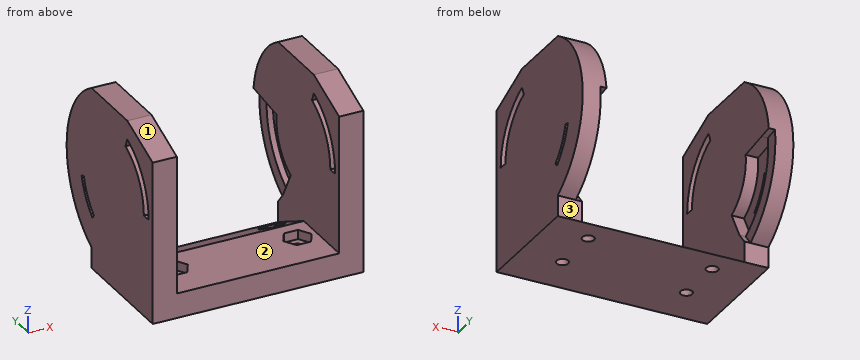
from build123d import *

# Parameters (mm, degrees)
CROQUIS1_W              = 34
CROQUIS1_H              = 19
SALIENTE_EXTRUIR1_DEPTH = 35
CROQUIS2_W              = 26.2
CROQUIS2_H              = 31
CORTAR_EXTRUIR1_DEPTH   = 25
CORTAR_EXTRUIR3_DEPTH   = 26.2
SALIENTE_EXTRUIR2_DEPTH = 34
CROQUIS10_W             = 26.2
CROQUIS10_H             = 25.966324345
CORTAR_EXTRUIR4_DEPTH   = 10
CORTAR_EXTRUIR5_START   = -34
CORTAR_EXTRUIR5_DEPTH   = 34
CORTAR_EXTRUIR6_DEPTH   = 2
CORTAR_EXTRUIR7_START   = 28.2
CORTAR_EXTRUIR7_DEPTH   = 28.2
CORTAR_EXTRUIR8_DEPTH   = 1
CORTAR_EXTRUIR9_DEPTH   = 27.2
CORTAR_EXTRUIR10_START  = -34
CORTAR_EXTRUIR10_DEPTH  = 34
CROQUIS18_R             = 0.95
CORTAR_EXTRUIR11_DEPTH  = 4
CORTAR_EXTRUIR12_DEPTH  = 1.5
CORTAR_EXTRUIR13_DEPTH  = 3


with BuildPart() as part:
    # Croquis1 → Saliente-Extruir1 (new body)
    with BuildSketch(Plane.XY):
        with Locations((-31.887263086, 5.12254902)):
            Rectangle(CROQUIS1_W, CROQUIS1_H)
    extrude(amount=SALIENTE_EXTRUIR1_DEPTH)

    # Croquis2 → Cortar-Extruir1 (cut)
    with BuildSketch(Plane.XZ.offset(4.37745098)):
        with Locations((-31.887263086, 19.5)):
            Rectangle(CROQUIS2_W, CROQUIS2_H)
    extrude(amount=-CORTAR_EXTRUIR1_DEPTH, mode=Mode.SUBTRACT)

    # Croquis4 → Cortar-Extruir3 (cut)
    with BuildSketch(Plane.ZY.offset(18.787263086)):
        Polygon((4, 14.62254902), (4, 6.62254902), (0, 14.62254902), align=None)
    extrude(amount=CORTAR_EXTRUIR3_DEPTH, mode=Mode.SUBTRACT)

    # Croquis9 → Saliente-Extruir2 (add)
    with BuildSketch(Plane(origin=(-14.887263086, 0, 0), x_dir=(0, 0, -1), z_dir=(1, 0, 0))):
        with BuildLine():
            Line((-29.315831827, 14.62254902), (-3.349507482, 14.62254902))
            ThreePointArc((-3.349507482, 14.62254902), (-16.332669655, 22.37254902), (-29.315831827, 14.62254902))
        make_face()
    extrude(amount=-SALIENTE_EXTRUIR2_DEPTH)

    # Croquis10 → Cortar-Extruir4 (cut)
    with BuildSketch(Plane.XZ.offset(-14.62254902)):
        with Locations((-31.887263086, 16.332669655)):
            Rectangle(CROQUIS10_W, CROQUIS10_H)
    extrude(amount=-CORTAR_EXTRUIR4_DEPTH, mode=Mode.SUBTRACT)

    # Croquis11 → Cortar-Extruir5 (cut)
    with BuildSketch(Plane(origin=(-14.887263086, 0, 0), x_dir=(0, 0, -1), z_dir=(1, 0, 0)).offset(CORTAR_EXTRUIR5_START)):
        with BuildLine():
            Line((-26.264575199, 3.509186373), (-24.878727914, 4.083143951))
            ThreePointArc((-24.878727914, 4.083143951), (-21.471881808, -0.068419609), (-16.332669655, -1.62745098))
            Line((-16.332669655, -1.62745098), (-16.332669655, -3.12745098))
            ThreePointArc((-16.332669655, -3.12745098), (-22.305267563, -1.31560371), (-26.264575199, 3.509186373))
        make_face()
        with BuildLine():
            Line((-13.621540157, 17.74062205), (-13.807242822, 17.04757027))
            ThreePointArc((-13.807242822, 17.04757027), (-11.089968726, 15.851941052), (-8.857991001, 13.894549121))
            Line((-8.857991001, 13.894549121), (-8.308354113, 14.355749231))
            ThreePointArc((-8.308354113, 14.355749231), (-10.704456257, 16.457074414), (-13.621540157, 17.74062205))
        make_face()
    extrude(amount=CORTAR_EXTRUIR5_DEPTH, mode=Mode.SUBTRACT)

    # Croquis12 → Cortar-Extruir6 (cut)
    with BuildSketch(Plane.ZY.offset(18.787263086)):
        with BuildLine():
            Line((17.258889566, 15.065137056), (17.873210354, 20.027255157))
            ThreePointArc((17.873210354, 20.027255157), (10.39091869, 18.620075808), (5.112868034, 13.133089064))
            Line((5.112868034, 13.133089064), (9.488064371, 10.688715764))
            ThreePointArc((9.488064371, 10.688715764), (12.652304566, 14.157448622), (17.258889566, 15.065137056))
        make_face()
    extrude(amount=-CORTAR_EXTRUIR6_DEPTH, mode=Mode.SUBTRACT)

    # Croquis14 → Cortar-Extruir7 (cut)
    with BuildSketch(Plane.ZY.offset(18.787263086).offset(CORTAR_EXTRUIR7_START)):
        with BuildLine():
            Line((17.873210354, 20.027255157), (17.258889566, 15.065137056))
            ThreePointArc((17.258889566, 15.065137056), (12.652304566, 14.157448622), (9.488064371, 10.688715764))
            Line((9.488064371, 10.688715764), (5.112868034, 13.133089064))
            ThreePointArc((5.112868034, 13.133089064), (10.39091869, 18.620075808), (17.873210354, 20.027255157))
        make_face()
    extrude(amount=-CORTAR_EXTRUIR7_DEPTH, mode=Mode.SUBTRACT)

    # Croquis15 → Cortar-Extruir8 (cut)
    with BuildSketch(Plane.ZY.offset(18.787263086)):
        with BuildLine():
            Line((17.873210354, 20.027255157), (18.15050768, 22.260102262))
            ThreePointArc((18.15050768, 22.260102262), (9.568856329, 20.730307382), (3.349507482, 14.62254902))
            Line((3.349507482, 14.62254902), (5.112868034, 13.133089064))
            ThreePointArc((5.112868034, 13.133089064), (10.39091869, 18.620075808), (17.873210354, 20.027255157))
        make_face()
    extrude(amount=-CORTAR_EXTRUIR8_DEPTH, mode=Mode.SUBTRACT)

    # Croquis15<2> → Cortar-Extruir9 (cut)
    with BuildSketch(Plane.ZY.offset(18.787263086)):
        with BuildLine():
            Line((17.873210354, 20.027255157), (18.15050768, 22.260102262))
            ThreePointArc((18.15050768, 22.260102262), (9.568856329, 20.730307382), (3.349507482, 14.62254902))
            Line((3.349507482, 14.62254902), (5.112868034, 13.133089064))
            ThreePointArc((5.112868034, 13.133089064), (10.39091869, 18.620075808), (17.873210354, 20.027255157))
        make_face()
    extrude(amount=CORTAR_EXTRUIR9_DEPTH, mode=Mode.SUBTRACT)

    # Croquis17 → Cortar-Extruir10 (cut)
    with BuildSketch(Plane(origin=(-14.887263086, 0, 0), x_dir=(0, 0, -1), z_dir=(1, 0, 0)).offset(CORTAR_EXTRUIR10_START)):
        Polygon((-29.315831827, 3.509186373), (-29.315831827, 14.62254902), (-35, 14.62254902), (-35, -4.37745098), (-26.264575199, -4.37745098), align=None)
    extrude(amount=CORTAR_EXTRUIR10_DEPTH, mode=Mode.SUBTRACT)

    # Croquis18 → Cortar-Extruir11 (cut)
    with BuildSketch(Plane(origin=(0, 0, 0), x_dir=(-1, 0, 0), z_dir=(0, 0, -1))):
        with Locations((41.887263086, 2.62254902)):
            Circle(CROQUIS18_R)
        with Locations((21.887263086, 2.62254902)):
            Circle(CROQUIS18_R)
        with Locations((21.887263086, 10.62254902)):
            Circle(CROQUIS18_R)
        with Locations((41.887263086, 10.62254902)):
            Circle(CROQUIS18_R)
    extrude(amount=-CORTAR_EXTRUIR11_DEPTH, mode=Mode.SUBTRACT)

    # Croquis19 → Cortar-Extruir12 (cut)
    with BuildSketch(Plane.XY.offset(4)):
        Polygon((-43.030772734, 0.616129568), (-40.721407694, 0.629030888), (-39.577898045, 2.63545034), (-40.743753437, 4.628968471), (-43.053118477, 4.616067151), (-44.196628126, 2.609647699), align=None)
        Polygon((-23.030772734, 0.616129568), (-20.721407694, 0.629030888), (-19.577898045, 2.63545034), (-20.743753437, 4.628968471), (-23.053118477, 4.616067151), (-24.196628126, 2.609647699), align=None)
    extrude(amount=-CORTAR_EXTRUIR12_DEPTH, mode=Mode.SUBTRACT)

    # Croquis20 → Cortar-Extruir13 (cut)
    with BuildSketch(Plane.XY.offset(4)):
        Polygon((-44.081159874, 10.610292765), (-42.973597252, 8.71645054), (-40.779700463, 8.728706795), (-39.520722563, 10.735771313), (-40.628285185, 12.629613538), (-42.994825708, 12.516391244), align=None)
        Polygon((-24.081159874, 10.610292765), (-22.973597252, 8.71645054), (-20.779700463, 8.728706795), (-19.520722563, 10.735771313), (-20.628285185, 12.629613538), (-22.994825708, 12.516391244), align=None)
    extrude(amount=-CORTAR_EXTRUIR13_DEPTH, mode=Mode.SUBTRACT)


solid = part.part
Work out the finished part from the listing and answer in its coordinate system (mm). Face numbers are marked on the shaded views. A direction names the side the tool comes from. Round coordinates to 2 decimals unless told otherwise and drop trailing zeros. Loops run counter-clockwise (first coordinate to the right, second up) from the corner with the lowest first, then second, coordinate; pieces in that order, holes last. Notation, with made-up numbers: (3, 79.5) - (9, 79.5) arc R22 cw to (9, 104.5) - close; hole circle Ø6 at (53.25, -5.5). An arc over 180 degrees is marked (long way). Use one line per item in the form item = value. Start each with the question number.
(1) Find section B-B on y = -0.5. Determine the outline of the cut face in (x, z).
(2) Find section D-D on y = 19.5. Determine the outline of the cut face in (x, z), and give its area (3 significant figures).
(3) Find section C-C on z = 22. Determine the outline of the cut face in (x, y), and give its area (3 significant figures).
(4) Find section A-A on z = 27.25. Determine the outline of the cut face in (x, y), and give its area (3 significant figures).
(5) Flat-ended cylindrical pins translate along their axes: P1, Ø2, axis at x = -42.5, y = 10, coming from the +Z side; P2, Ø1.5, axis at x = -41.89, y = 10.62, coming from the -Z side; P3, Ø2, axis at x = -42, y = 3, coming from the +Z side; P4, Ø8, axis at x = -34, z = 4.5, coming from the +Y side. Find the tip coordinate at first contact, or state that the pin passes through.
(6) Which of the six approach directions +Z, -Z, +X, -X, +Y, -Y give full straight-line access (tool end or side, diameter ignored) to the marked faces 1, 2 and 3?
(7) Consider line 1 (X direction, y = 9.25, z = 27.25); line 2 (X direction, y = 19.75, z = 8); line 3 (Y direction, x = -45.5, z = 16.5). Determine where each line is inside the solid, lowest interval first.
Answer list:
q1.outline = (-48.89, 0) - (-14.89, 0) - (-14.89, 20.76) - (-18.79, 20.76) - (-18.79, 4) - (-44.99, 4) - (-44.99, 20.76) - (-48.89, 20.76) - close; (-48.89, 23.37) - (-44.99, 23.37) - (-44.99, 27.76) - (-48.89, 27.76) - close; (-18.79, 23.37) - (-14.89, 23.37) - (-14.89, 27.76) - (-18.79, 27.76) - close
q2.outline = (-48.89, 7.59) - (-45.99, 7.59) - (-45.99, 12.44) - (-46.99, 12.44) - (-46.99, 17.81) - (-44.99, 17.81) - (-44.99, 25.08) - (-48.89, 25.08) - close; (-18.79, 17.81) - (-16.79, 17.81) - (-16.79, 12.44) - (-17.79, 12.44) - (-17.79, 7.59) - (-14.89, 7.59) - (-14.89, 25.08) - (-18.79, 25.08) - close
q2.area = 105 mm^2
q3.outline = (-48.89, -4.38) - (-44.99, -4.38) - (-44.99, -1.51) - (-48.89, -1.51) - close; (-48.89, 0.31) - (-44.99, 0.31) - (-44.99, 21.24) - (-48.89, 21.24) - close; (-18.79, -4.38) - (-14.89, -4.38) - (-14.89, -1.51) - (-18.79, -1.51) - close; (-18.79, 0.31) - (-14.89, 0.31) - (-14.89, 21.24) - (-18.79, 21.24) - close
q3.area = 186 mm^2
q4.outline = (-48.89, -1.83) - (-44.99, -1.83) - (-44.99, 17.54) - (-48.89, 17.54) - close; (-18.79, -1.83) - (-14.89, -1.83) - (-14.89, 17.54) - (-18.79, 17.54) - close
q4.area = 151 mm^2
q5.P1 = 1
q5.P2 = through
q5.P3 = 2.5
q5.P4 = 13.62
q6.face_1 = +Z, +X, -X, -Y
q6.face_2 = +Z, +Y, -Y
q6.face_3 = -Z, +X, -X, +Y
q7.line_1 = -48.89 to -44.99, -18.79 to -14.89
q7.line_2 = -48.89 to -45.99, -17.79 to -14.89
q7.line_3 = -4.38 to -3.13, -1.63 to 15.12
